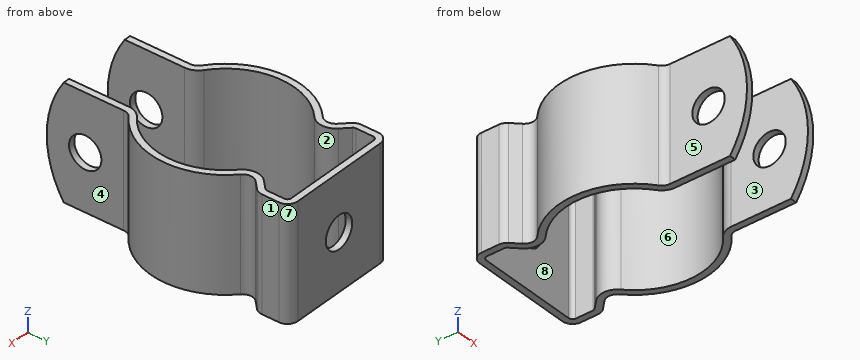
```python
from build123d import *

# Parameters (mm, degrees)
BOSS_EXTRUDE1_DEPTH      = 11.1125
BOSS_EXTRUDE1_DEPTH_BACK = 11.1125
SKETCH4_R                = 3.175
CUT_EXTRUDE1_DEPTH       = 22.225
CUT_EXTRUDE2_DEPTH       = 35.029202096
CUT_EXTRUDE2_DEPTH_BACK  = 35.029202096
CUT_EXTRUDE3_DEPTH       = 35.029202096
CUT_EXTRUDE3_DEPTH_BACK  = 35.029202096
SKETCH6_R                = 3.175


with BuildPart() as part:
    # Sketch3 → Boss-Extrude1 (new, two sides: drawn at the far end of the back side and taken through both)
    with BuildSketch(Plane.XY.offset(-BOSS_EXTRUDE1_DEPTH_BACK)):
        with BuildLine():
            Line((-10.668, 16.843375), (-10.668, 20.193))
            ThreePointArc((-10.668, 20.193), (-10.444815367, 20.731815367), (-9.906, 20.955))
            Line((-9.906, 20.955), (9.906, 20.955))
            ThreePointArc((9.906, 20.955), (10.444815367, 20.731815367), (10.668, 20.193))
            Line((10.668, 20.193), (10.668, 16.843375))
            ThreePointArc((10.668, 16.843375), (10.609996204, 16.551770225), (10.444815367, 16.304559633))
            Line((10.444815367, 16.304559633), (8.931602372, 14.791346638))
            ThreePointArc((8.931602372, 14.791346638), (7.965505779, 12.373739179), (9.051510982, 10.007569035))
            ThreePointArc((9.051510982, 10.007569035), (13.477623457, -0.659511197), (8.031189621, -10.84349032))
            ThreePointArc((8.031189621, -10.84349032), (7.047523696, -12.011383636), (6.694468964, -13.496956187))
            Line((6.694468964, -13.496956187), (6.694468964, -28.575))
            Line((6.694468964, -28.575), (7.964468964, -28.575))
            Line((7.964468964, -28.575), (7.964468964, -13.496956187))
            ThreePointArc((7.964468964, -13.496956187), (8.181733414, -12.582757694), (8.787066292, -11.864054115))
            ThreePointArc((8.787066292, -11.864054115), (14.746105665, -0.721582839), (9.903417898, 10.949457886))
            ThreePointArc((9.903417898, 10.949457886), (9.235107004, 12.40556259), (9.829627985, 13.893321026))
            Line((9.829627985, 13.893321026), (11.342840979, 15.406534021))
            ThreePointArc((11.342840979, 15.406534021), (11.78332321, 16.065762265), (11.938, 16.843375))
            Line((11.938, 16.843375), (11.938, 20.193))
            ThreePointArc((11.938, 20.193), (11.342840979, 21.629840979), (9.906, 22.225))
            Line((9.906, 22.225), (-9.906, 22.225))
            ThreePointArc((-9.906, 22.225), (-11.342840979, 21.629840979), (-11.938, 20.193))
            Line((-11.938, 20.193), (-11.938, 16.843375))
            ThreePointArc((-11.938, 16.843375), (-11.78332321, 16.065762265), (-11.342840979, 15.406534021))
            Line((-11.342840979, 15.406534021), (-9.829627985, 13.893321026))
            ThreePointArc((-9.829627985, 13.893321026), (-9.235107004, 12.40556259), (-9.903417898, 10.949457886))
            ThreePointArc((-9.903417898, 10.949457886), (-14.746105665, -0.721582839), (-8.787066292, -11.864054115))
            ThreePointArc((-8.787066292, -11.864054115), (-8.181733414, -12.582757694), (-7.964468964, -13.496956187))
            Line((-7.964468964, -13.496956187), (-7.964468964, -28.575))
            Line((-7.964468964, -28.575), (-6.694468964, -28.575))
            Line((-6.694468964, -28.575), (-6.694468964, -13.496956187))
            ThreePointArc((-6.694468964, -13.496956187), (-7.047523696, -12.011383636), (-8.031189621, -10.84349032))
            ThreePointArc((-8.031189621, -10.84349032), (-13.477623457, -0.659511197), (-9.051510982, 10.007569035))
            ThreePointArc((-9.051510982, 10.007569035), (-7.965505779, 12.373739179), (-8.931602372, 14.791346638))
            Line((-8.931602372, 14.791346638), (-10.444815367, 16.304559633))
            ThreePointArc((-10.444815367, 16.304559633), (-10.609996204, 16.551770225), (-10.668, 16.843375))
        make_face()
    extrude(amount=BOSS_EXTRUDE1_DEPTH + BOSS_EXTRUDE1_DEPTH_BACK)

    # Sketch4 → Cut-Extrude1 (cut)
    with BuildSketch(Plane(origin=(0, 22.225, 0), x_dir=(1, 0, 0), z_dir=(0, 1, 0))):
        with Locations(Location((0, 0, 0), (0, 0, 270))):
            Circle(SKETCH4_R)
    extrude(amount=-CUT_EXTRUDE1_DEPTH, mode=Mode.SUBTRACT)

    # Sketch5 → Cut-Extrude2 (cut, two sides: drawn at the far end of the back side and taken through both)
    with BuildSketch(Plane(origin=(0, 0, 0), x_dir=(0, 0, -1), z_dir=(1, 0, 0)).offset(-CUT_EXTRUDE2_DEPTH_BACK)):
        with BuildLine():
            Line((-11.1125, -25.24125), (-11.1125, -31.90875))
            Line((-11.1125, -31.90875), (11.1125, -31.90875))
            Line((11.1125, -31.90875), (11.1125, -25.24125))
            ThreePointArc((11.1125, -25.24125), (0, -28.575), (-11.1125, -25.24125))
        make_face()
    extrude(amount=CUT_EXTRUDE2_DEPTH + CUT_EXTRUDE2_DEPTH_BACK, mode=Mode.SUBTRACT)

    # Sketch6 → Cut-Extrude3 (cut, two sides: drawn at the far end of the back side and taken through both)
    with BuildSketch(Plane(origin=(0, 0, 0), x_dir=(0, 0, -1), z_dir=(1, 0, 0)).offset(-CUT_EXTRUDE3_DEPTH_BACK)):
        with Locations(Location((0, -21.035978094, 0), (0, 0, 270))):
            Circle(SKETCH6_R)
    extrude(amount=CUT_EXTRUDE3_DEPTH + CUT_EXTRUDE3_DEPTH_BACK, mode=Mode.SUBTRACT)


solid = part.part
```
The listing builds one solid part. Answer for the finished solid, in the listing's coordinates (mm). Face numbers are marked on the shaded views. A direction names the side the tool comes from. Coordinates: 2 decimals unless noted, no trailing zeros. Write each loop counter-clockwise with the first axis right and the second up, starting at its lowest first coordinate (ties: lowest second). Pieces come first, ordered by that corner, then holes. Notation, with made-up numbers: (5.25, 14.5) -> (63.25, 14.5) arc R15 ccw to (63.25, 26.5) -> close; hole circle Ø8 at (63, -6.5). An arc over 180 degrees is marked (long way). Write each question's results on one line, items separated by ' | '. Start each with the question number.
1) A cutting plane is placed at C-C (x = 0). Determine the outline of the cut face in (y, z) (1 decimal).
2) For a pull along Y with two mould halves and no side action, classify the marked faces 5, 6, 7 and 8 as +Y half, -Y half, draft (parallel to the pull), parting line (faces both ways), or undercut.
3) Straight lines are drawn through the part: probe 1 along X at (y, z) = (-23, -3); probe 2 along X at (y, z) = (17.5, -9.5); probe 3 along Y at (x, z) = (-6, -7.25) (3 decimals). For each, find the intervals that lie inside material, in ascending order.
4) A cutting plane is placed at A-A (x = 7.25). Count the separate pieces of the cut face and the enclosed holes in it, then the cut area to 3 significant figures.
5) A cutting plane is placed at B-B (y = 1). Determine the outline of the cut face in (x, z).
6) A tool of negligible diameter and unlimited length cuts with its end or side. For the marked faces 1, 2, 3 and 4, from which of +Z, -Z, +X, -X, +Y, -Y can it reach the whole face along a straight path? Write none if from no direction.
7) Flat-ended cylindrical pins translate along their axes: pin 1 Ø1.7 at (y, z) = (19, 1.5) entering from +X; pin 2 Ø7.5 at (y, z) = (-24, -1.5) entering from +X; pin 3 Ø2 at (y, z) = (2.5, -3.5) entering from -X. Find the tip coordinate at first contact, or state that the pin passes through.
Values follow:
1) outline: (21, -11.1) -> (22.2, -11.1) -> (22.2, -3.2) -> (21, -3.2) -> close; (21, 3.2) -> (22.2, 3.2) -> (22.2, 11.1) -> (21, 11.1) -> close
2) face 5: draft | face 6: undercut | face 7: +Y half | face 8: undercut
3) probe 1: -7.96 to -6.69, 6.69 to 7.96 | probe 2: -11.94 to -10.67, 10.67 to 11.94 | probe 3: 20.955 to 22.225
4) separate pieces: 2 | enclosed holes: 1 | area: 349 mm²
5) outline: (-14.73, -11.11) -> (-13.46, -11.11) -> (-13.46, 11.11) -> (-14.73, 11.11) -> close; (13.46, -11.11) -> (14.73, -11.11) -> (14.73, 11.11) -> (13.46, 11.11) -> close
6) face 1: +Z, -Z, +X, +Y | face 2: +Z, -Z | face 3: +Z, -Z, -Y | face 4: +Z, -Z, +X, -Y
7) pin 1: x = 11.94 | pin 2: x = 7.96 | pin 3: x = -14.69
